Geometry: final body of the model. Coordinates: model frame, mm. A direction names the side the tool comes from. Coordinates: 2 decimals unless noted, no trailing zeros. Loops run counter-clockwise (first coordinate to the right, second up) from the corner with the lowest first, then second, coordinate; pieces in that order, holes last. Notation, with made-up numbers: (49, 26) - (88, 26) arc R11 ccw to (88, 33) - close; hole circle Ø4 at (5.25, -6.5). An arc over 180 degrees is marked (long way). Answer in a Markdown table with one row per item.
from build123d import *

# Parameters (mm, degrees)
SKETCH_2_R          = 1.75
CUT_EXTRUDE_1_DEPTH = 12
SKETCH_3_R          = 1.75
CUT_EXTRUDE_2_DEPTH = 12
CUT_EXTRUDE_5_DEPTH = 6


with BuildPart() as part:
    # 草图1 → 旋转1 (revolve)
    with BuildSketch(Plane(origin=(0, 0, 0), x_dir=(1, 0, 0), z_dir=(0, 1, 0)), mode=Mode.PRIVATE) as revolve_1_sk:
        Polygon((-41.4, 0.193025833), (-41.4, 4.193025833), (0, 4.193025833), (0, 12.693025833), (6, 12.693025833), (6, 4.193025833), (34, 4.193025833), (34, 0.193025833), align=None)
    revolve(revolve_1_sk.sketch.rotate(Axis((-41.4, 0, -0.193025833), (1, 0, 0)), 180), axis=Axis((-41.4, 0, -0.193025833), (1, 0, 0)))

    # 草图2 → 拉伸1 (cut)
    with BuildSketch(Plane(origin=(34, 0, 0), x_dir=(0, 0, -1), z_dir=(1, 0, 0))):
        Circle(SKETCH_2_R)
    extrude(amount=-CUT_EXTRUDE_1_DEPTH, mode=Mode.SUBTRACT)

    # 草图3 → 拉伸2 (cut)
    with BuildSketch(Plane.ZY.offset(41.4)):
        with Locations((-0.193025833, 0)):
            Circle(SKETCH_3_R)
    extrude(amount=-CUT_EXTRUDE_2_DEPTH, mode=Mode.SUBTRACT)

    # 草图4 → 拉伸5 (cut, symmetric)
    with BuildSketch(Plane.XY):
        Polygon((-41.4, 4), (-41.4, 3), (-38.2827279, 3), (-37.855795833, 4), align=None)
        Polygon((34, 4), (30.455795833, 4), (30.8827279, 3), (34, 3), align=None)
        Polygon((-41.4, -4), (-41.4, -3), (-38.2827279, -3), (-37.855795833, -4), align=None)
        Polygon((30.8827279, -3), (34, -3), (34, -4), (30.455795833, -4), align=None)
    extrude(amount=CUT_EXTRUDE_5_DEPTH, both=True, mode=Mode.SUBTRACT)


solid = part.part
(1) Cut plane A-A on y = 0. Output: boundary loops of the cut face in (x, z).
Verdict:
| item | result |
|---|---|
| outline | (-41.4, -4.19) - (0, -4.19) - (0, -12.69) - (6, -12.69) - (6, -4.19) - (34, -4.19) - (34, -1.75) - (22, -1.75) - (22, 1.75) - (34, 1.75) - (34, 3.81) - (6, 3.81) - (6, 12.31) - (0, 12.31) - (0, 3.81) - (-41.4, 3.81) - (-41.4, 1.56) - (-29.4, 1.56) - (-29.4, -1.94) - (-41.4, -1.94) - close |
(2) Ray query, probe 1 along Y at (x, z) = (28.75, 0); probe 2 along X at (y, z) = (-3.5, 3.5); probe 3 along Y at (x, z) = (-5.5, -3.5). Return the intervals inside material, ascending.
Verdict:
| item | result |
|---|---|
| probe 1 | y = -4 to -1.75, 1.75 to 4 |
| probe 2 | x = 0 to 6 |
| probe 3 | y = -2.25 to 2.25 |
(3) First-contact query: pin 1 Ø1.5 at (x, z) = (-21.5, 2) entering from -Y; pin 2 Ø3 at (x, z) = (-10.5, 2) entering from +Y; pin 3 Ø5 at (y, z) = (7.5, -2) entering from +X. Flat tips, straight axial feed; report the tip coordinate or a pass-through.
Verdict:
| item | result |
|---|---|
| pin 1 | stops at y = -3.73 |
| pin 2 | stops at y = 3.94 |
| pin 3 | stops at x = 6 |
(4) Cut plane D-D on x = -24.5. Output: boundary loops of the cut face in (y, z).
Verdict:
| item | result |
|---|---|
| outline | circle Ø8 at (0, -0.19) |
(5) Access query for faces 4 (the face through (28.084, -0.67, -1.617)), 5 (the face through (-40, 3, 0)), 6 (the face through (-29.4, 0, 0)), 7 (the face through (32, -3, 0)), 8 (the face through (34, 0, -2)). Directions: +Z, -Z, +X, -X, +Y, -Y. A direction counts if a zero-diameter tool reaches every point of the face in a straight line with its end or side. Return the directions, or none.
Verdict:
| item | result |
|---|---|
| face 4 | +X |
| face 5 | +Z, -Z, -X, +Y |
| face 6 | -X |
| face 7 | +Z, -Z, +X, -Y |
| face 8 | +Z, -Z, +X, +Y, -Y |
(6) Cut plane C-C on z = -8. Output: boundary loops of the cut face in (x, y), then the cut area to 3 significant figures.
Verdict:
| item | result |
|---|---|
| outline | (0, -9.76) - (6, -9.76) - (6, 9.76) - (0, 9.76) - close |
| area | 117 mm² |
(7) Pull-direction query (Y, two-part tool) for faces 1 (the face through (-35.484, -0.67, 1.424)), 2 (the face through (32, 3, 0)), 3 (the face through (-40, -3, 0)); classes: pulls with the +Y half, pulls with the -Y half, needs draft (parallel to the pull), parting line crosses it, or undercut.
Verdict:
| item | result |
|---|---|
| face 1 | undercut |
| face 2 | pulls with the +Y half |
| face 3 | pulls with the -Y half |
(8) Cut plane B-B on x = 28. Output: boundary loops of the cut face in (y, z).
Verdict:
| item | result |
|---|---|
| outline | circle Ø8 at (0, -0.19); hole circle Ø3.5 at (0, 0) |
